from build123d import *

# Parameters (mm, degrees)
SKETCH1_W           = 45.5
SKETCH1_H           = 124.4
BOSS_EXTRUDE1_DEPTH = 1.2
SKETCH2_W           = 5
SKETCH2_H           = 11.428571429
CUT_EXTRUDE1_DEPTH  = 1.6
FILLET1_R           = 2
FILLET2_R           = 1
FILLET3_R           = 5


with BuildPart() as part:
    # Sketch1 → Boss-Extrude1 (new body)
    with BuildSketch(Plane.XY):
        with Locations((22.75, 62.2)):
            Rectangle(SKETCH1_W, SKETCH1_H)
    extrude(amount=BOSS_EXTRUDE1_DEPTH)

    # Sketch2 → Cut-Extrude1 (cut)
    with BuildSketch(Plane.XY.offset(1.2)):
        Polygon((14, 82.2), (19, 82.2), (19, 86.2), (10, 86.2), (10, 70.771428571), (14, 70.771428571), align=None)
        with Locations((16.5, 76.485714285)):
            Rectangle(SKETCH2_W, SKETCH2_H)
        Polygon((26.5, 70.771428571), (26.5, 82.2), (19, 82.2), (19, 70.771428571), (14, 70.771428571), (14, 53.628571429), (19, 53.628571429), (19, 42.2), (26.5, 42.2), (26.5, 53.628571429), (31.5, 53.628571429), (31.5, 70.771428571), align=None)
        with Locations((29, 76.485714285)):
            Rectangle(SKETCH2_W, SKETCH2_H)
        Polygon((35.5, 70.771428571), (35.5, 86.2), (26.5, 86.2), (26.5, 82.2), (31.5, 82.2), (31.5, 70.771428571), align=None)
        Polygon((35.5, 53.628571429), (31.5, 53.628571429), (31.5, 42.2), (26.5, 42.2), (26.5, 38.2), (35.5, 38.2), align=None)
        with Locations((29, 47.914285715)):
            Rectangle(SKETCH2_W, SKETCH2_H)
        Polygon((14, 42.2), (14, 53.628571429), (10, 53.628571429), (10, 38.2), (19, 38.2), (19, 42.2), align=None)
        with Locations((16.5, 47.914285715)):
            Rectangle(SKETCH2_W, SKETCH2_H)
    extrude(amount=-CUT_EXTRUDE1_DEPTH, mode=Mode.SUBTRACT)

    # Fillet1
    fillet1_edges = [part.edges().sort_by_distance(p)[0] for p in [
        (10, 70.771428571, 0.6),
        (19, 86.2, 0.6),
        (26.5, 86.2, 0.6),
        (35.5, 86.2, 0.6),
        (35.5, 70.771428571, 0.6),
        (31.5, 70.771428571, 0.6),
        (31.5, 53.628571429, 0.6),
        (35.5, 53.628571429, 0.6),
        (35.5, 38.2, 0.6),
        (26.5, 38.2, 0.6),
        (19, 38.2, 0.6),
        (10, 38.2, 0.6),
        (10, 53.628571429, 0.6),
        (14, 53.628571429, 0.6),
        (14, 70.771428571, 0.6),
        (10, 86.2, 0.6),
    ]]
    fillet(fillet1_edges, radius=FILLET1_R - 0.0001)  # a hair under: the kernel refuses the full size

    # Fillet2
    fillet2_edges = [part.edges().sort_by_distance(p)[0] for p in [
        (19, 42.2, 0.6),
        (19, 82.2, 0.6),
        (26.5, 82.2, 0.6),
        (26.5, 42.2, 0.6),
    ]]
    fillet(fillet2_edges, radius=FILLET2_R)

    # Fillet3
    fillet3_edges = [part.edges().sort_by_distance(p)[0] for p in [
        (0, 124.4, 0.6),
        (45.5, 124.4, 0.6),
        (45.5, 0, 0.6),
        (0, 0, 0.6),
    ]]
    fillet(fillet3_edges, radius=FILLET3_R)


solid = part.part
The listing builds one solid part. Answer for the finished solid, in the listing's coordinates (mm). A direction names the side the tool comes from. Coordinates: 2 decimals unless noted, no trailing zeros. Order: outer loops, then holes, each group sorted by start corner. A loop starts at its lowest first (then second) coordinate and runs counter-clockwise, first axis right, second up. Notation, with made-up numbers: M 68.5,-5.75 L 119.5,-5.75 A25 ccw 119.5,20.25 Z; hole C -13,45.5 d10. An arc over 180 degrees is marked long. Use CSV: the item, a comma, the result in double quotes.
Q1. Section A-A (x = 24) is taken. Determine the outline of the cut face in (y, z).
Here are the results:
outline,"M 0,0 L 42.2,0 L 42.2,1.2 L 0,1.2 Z; M 82.2,0 L 124.4,0 L 124.4,1.2 L 82.2,1.2 Z"
Q2. Straight lines are drawn through the part: L1, parallel to X at y = 78.5, z = 0.1; L2, parallel to Y at x = 25.5, z = 0.4; L3, parallel to Y at x = 11.5, z = 1.15. For each, find the intervals that lie inside material, in ascending order.
Here are the results:
L1,"0 to 10, 35.5 to 45.5"
L2,"0 to 42.2, 82.2 to 124.4"
L3,"0 to 38.26, 53.57 to 70.83, 86.14 to 124.4"
Q3. A tool of negligible diameter and unlimited length cuts with its end or side. For faces 1 (the flat face through (33, 63, 1.2)), 2 (the cylindrical face through (10.57, 71.373, 0.592)), from which of +Z, -Z, +X, -X, +Y, -Y can it reach the whole face along a straight path? Write none if from no direction.
Here are the results:
face 1,"+Z, +X, -X, +Y, -Y"
face 2,"+Z, -Z"
Q4. Section B-B (y = 58) is taken. Determine the outline of the cut face in (x, z).
Here are the results:
outline,"M 0,0 L 14,0 L 14,1.2 L 0,1.2 Z; M 31.5,0 L 45.5,0 L 45.5,1.2 L 31.5,1.2 Z"
Q5. Determine the mould class of faces 3 (the cylindrical face through (1, 2, 1)), 4 (the cylindrical face through (27.1, 85.63, 0.59)), 5 (the flat face through (33, 63, 0)) for opening direction Y: pulls with the +Y half, pulls with the -Y half, needs draft (parallel to the pull), parting line crosses it, or undercut.
Here are the results:
face 3,"pulls with the -Y half"
face 4,"undercut"
face 5,"needs draft"
